```python
from build123d import *

# Parameters (mm, degrees)
SKETCH_3_R          = 12.5
CUT_EXTRUDE_1_DEPTH = 164.157898981


with BuildPart() as part:
    # 草圖2 → 旋轉1 (revolve)
    with BuildSketch(Plane.XY, mode=Mode.PRIVATE) as revolve_1_sk:
        Polygon((0, 0), (0, 20), (89, 20), (89, 5), (114.5, 5), (114.5, 0), align=None)
    revolve(revolve_1_sk.sketch.rotate(Axis((0, 0, 0), (0, 1, 0)), 90), axis=Axis((0, 0, 0), (0, 1, 0)))

    # 草圖3 → 除料-伸長1 (cut, through all)
    with BuildSketch(Plane(origin=(0, 20, 0), x_dir=(1, 0, 0), z_dir=(0, 1, 0))):
        with Locations(Location((0, 63.124852982, 0), (0, 0, 270))):
            Circle(SKETCH_3_R)
        with Locations(Location((63.124852982, 0, 0), (0, 0, 270))):
            Circle(SKETCH_3_R)
        with Locations(Location((0, -63.124852982, 0), (0, 0, 270))):
            Circle(SKETCH_3_R)
        with Locations(Location((-63.124852982, 0, 0), (0, 0, 270))):
            Circle(SKETCH_3_R)
    extrude(amount=-CUT_EXTRUDE_1_DEPTH, mode=Mode.SUBTRACT)


solid = part.part
```
Part model, mm, in its own coordinate system. A direction names the side the tool comes from. Round coordinates to 2 decimals unless told otherwise and drop trailing zeros. Loops run counter-clockwise (first coordinate to the right, second up) from the corner with the lowest first, then second, coordinate; pieces in that order, holes last.
Item 1: Mould opens along Z. For faces 3 (the face through (67, 5, 59)), 4 (the face through (111.777, 2.465, 24.821)), 5 (the face through (3.75, 10.14, 75.05)) say: +Z half, -Z half, draft (parallel to the pull), parting line (faces both ways), or undercut.
Item 2: Drop flat-ended pins along their axis: P1, Ø1.5, axis at x = -62.5, z = 76, coming from the -Y side; P2, Ø2, axis at x = -83.5, y = 16, coming from the -Z side; P3, Ø10, axis at y = 14, z = -35.5, coming from the -X side; P4, Ø1.5, axis at x = 14, y = 16, coming from the +Z side. Give the stop position or say it passes through.
Item 3: 3-axis set-ups, long thin cutter, end or side, ignore diameter. For faces 1 (the face through (-60.15, 12.395, 65.597)), 2 (the face through (-2, 0, 2)): which of +Z, -Z, +X, -X, +Y, -Y reach the whole face in a straight line?
Item 4: Drill centre lines: line 1 (X direction, y = 6.5, z = 0); line 2 (Z direction, x = -72, y = 6.5); line 3 (Y direction, x = -101, z = 25). Where is each one in solid material? Low to high.
Item 5: Cut at C-C, the plane x = -53.5. Give the cut face in (y, z), then the cut area to 3 significant figures.
Item 6: Cut at B-B, the plane z = 0. Give the cut face in (x, y).
Item 7: Cut at D-D, the plane y = 10.25. Give the cut face in (x, z).
Item 8: Cut at A-A, the plane x = 0. Give the cut face in (y, z).
A:
1. face 3: draft
1. face 4: parting line
1. face 5: undercut
2. P1: stops at y = 0
2. P2: stops at z = -33.39
2. P3: stops at x = -83.61
2. P4: stops at z = 88.01
3. face 1: +Y
3. face 2: +Z, -Z, +X, -X, -Y
4. line 1: x = -89 to -75.62, -50.62 to 50.62, 75.62 to 89
4. line 2: z = -52.32 to -8.8, 8.8 to 52.32
4. line 3: y = 0 to 5
5. outline: (0, -101.23) - (5, -101.23) - (5, -71.12) - (20, -71.12) - (20, -7.98) - (0, -7.98) - close; (0, 7.98) - (20, 7.98) - (20, 71.12) - (5, 71.12) - (5, 101.23) - (0, 101.23) - close
5. area: 2,830 mm2
6. outline: (-114.5, 0) - (-75.62, 0) - (-75.62, 20) - (-89, 20) - (-89, 5) - (-114.5, 5) - close; (-50.62, 0) - (50.62, 0) - (50.62, 20) - (-50.62, 20) - close; (75.62, 0) - (114.5, 0) - (114.5, 5) - (89, 5) - (89, 20) - (75.62, 20) - close
7. outline: circle Ø178 at (0, 0); hole circle Ø25 at (-63.12, 0); hole circle Ø25 at (0, -63.12); hole circle Ø25 at (0, 63.12); hole circle Ø25 at (63.12, 0)
8. outline: (0, -114.5) - (5, -114.5) - (5, -89) - (20, -89) - (20, -75.62) - (0, -75.62) - close; (0, -50.62) - (20, -50.62) - (20, 50.62) - (0, 50.62) - close; (0, 75.62) - (20, 75.62) - (20, 89) - (5, 89) - (5, 114.5) - (0, 114.5) - close
